from build123d import *

# Parameters (mm, degrees)
SKETCH1_W           = 120
SKETCH1_H           = 42
SKETCH1_R           = 1.5
SKETCH1_R_2         = 3.4
SKETCH1_W_2         = 10
SKETCH1_H_2         = 3
SKETCH1_W_3         = 40
SKETCH1_H_3         = 16
BOSS_EXTRUDE1_DEPTH = 3


with BuildPart() as part:
    # Sketch1 → Boss-Extrude1 (new body)
    with BuildSketch(Plane(origin=(0, 0, 0), x_dir=(0, 0, -1), z_dir=(1, 0, 0))):
        Rectangle(SKETCH1_W, SKETCH1_H)
        with Locations((49, 9)):
            Circle(SKETCH1_R, mode=Mode.SUBTRACT)
        with Locations((13, 9)):
            Circle(SKETCH1_R, mode=Mode.SUBTRACT)
        with Locations((-14.5, -0.4)):
            Circle(SKETCH1_R_2, mode=Mode.SUBTRACT)
        with Locations((57.5, 0)):
            Circle(SKETCH1_R, mode=Mode.SUBTRACT)
        with Locations((-57.5, 0)):
            Circle(SKETCH1_R, mode=Mode.SUBTRACT)
        with Locations((25, -18.5)):
            Rectangle(SKETCH1_W_2, SKETCH1_H_2, mode=Mode.SUBTRACT)
        with Locations((-25, -18.5)):
            Rectangle(SKETCH1_W_2, SKETCH1_H_2, mode=Mode.SUBTRACT)
        with Locations((25, 18.5)):
            Rectangle(SKETCH1_W_2, SKETCH1_H_2, mode=Mode.SUBTRACT)
        with Locations((-25, 18.5)):
            Rectangle(SKETCH1_W_2, SKETCH1_H_2, mode=Mode.SUBTRACT)
        with Locations((31, -4)):
            Rectangle(SKETCH1_W_3, SKETCH1_H_3, mode=Mode.SUBTRACT)
    extrude(amount=BOSS_EXTRUDE1_DEPTH)


solid = part.part
Work out the finished part from the listing and answer in its coordinate system (mm). A direction names the side the tool comes from. Round coordinates to 2 decimals unless told otherwise and drop trailing zeros. Order: outer loops, then holes, each group sorted by start corner. A loop starts at its lowest first (then second) coordinate and runs counter-clockwise, first axis right, second up. Notation, with made-up numbers: M 29,2.25 L 78,2.25 A26 ccw 78,23.25 Z; hole C -28,-24 d9. An arc over 180 degrees is marked long. Put each result on its own line as item: value. Start each with the question number.
Q1. Section C-C, the plane z = 24.5 is taken. Write down the section's boundary in (x, y).
Q2. Straight lines are drawn through the part: L1, parallel to Y at x = 1.6, z = -49; L2, parallel to Y at x = 0.25, z = 29.5; L3, parallel to Y at x = 1.95, z = -45.5. For each, find the intervals that lie inside material, in ascending order. Write a range as [from, to].
Q3. A flat-ended cylindrical pin translates along its axis: pin 1 (2.5 mm diameter, centred on y = 9, z = -49, fed in from +X). Find the tip coordinate at first contact, or state that the pin passes through.
Q4. For a pull along Z with two mould halves and no side action, classify faces 3 (the flat face through (0, 0, 1)), 4 (the flat face through (1, -19, -30)), 5 (the flat face through (1, 0, -60)) as pulls with the +Z half, pulls with the -Z half, needs draft (parallel to the pull), parting line crosses it, or undercut.
Q5. A tool of negligible diameter and unlimited length cuts with its end or side. For faces 1 (the flat face through (1, 4, -31)), 2 (the flat face through (1, 21, 1)), from which of +Z, -Z, +X, -X, +Y, -Y can it reach the whole face along a straight path? Write none if from no direction.
Q6. Section B-B, the plane z = 57.5 is taken. Write down the section's boundary in (x, y), and give its area (3 significant figures).
Q7. Section D-D, the plane y = -7.5 is taken. Write down the section's boundary in (x, z), and give its area (3 significant figures).
Q8. Section A-A, the plane y = 9 is taken. Write down the section's boundary in (x, z).
Findings below:
1. outline: M 0,-21 L 3,-21 L 3,-20 L 0,-20 Z; M 0,-17 L 3,-17 L 3,17 L 0,17 Z; M 0,20 L 3,20 L 3,21 L 0,21 Z
2. L1: y = [-21, -12], [4, 7.5], [10.5, 21]
2. L2: y = [-21, -20], [-17, 17], [20, 21]
2. L3: y = [-21, -12], [4, 21]
3. pin 1: passes through
4. face 3: needs draft
4. face 4: undercut
4. face 5: pulls with the -Z half
5. face 1: +X, -X
5. face 2: +Z, -Z, +X, -X, +Y
6. outline: M 0,-21 L 3,-21 L 3,-1.5 L 0,-1.5 Z; M 0,1.5 L 3,1.5 L 3,21 L 0,21 Z
6. area: 117 mm^2
7. outline: M 0,-60 L 3,-60 L 3,-51 L 0,-51 Z; M 0,-11 L 3,-11 L 3,60 L 0,60 Z
7. area: 240 mm^2
8. outline: M 0,-60 L 3,-60 L 3,-50.5 L 0,-50.5 Z; M 0,-47.5 L 3,-47.5 L 3,-14.5 L 0,-14.5 Z; M 0,-11.5 L 3,-11.5 L 3,60 L 0,60 Z
